from build123d import *

# Parameters (mm, degrees)
BOSS_EXTRUDE1_DEPTH = 35.687
SKETCH2_R           = 4.1656
CUT_EXTRUDE1_DEPTH  = 77.2
SKETCH3_R           = 4.1656
CUT_EXTRUDE2_DEPTH  = 77.2


with BuildPart() as part:
    # Sketch1 → Boss-Extrude1 (new body, symmetric)
    with BuildSketch(Plane.XY):
        with BuildLine():
            Line((0, 0), (0, 76.2))
            ThreePointArc((0, 76.2), (4.490128061, 74.340128061), (6.35, 69.85))
            Line((6.35, 69.85), (6.35, 14.2748))
            ThreePointArc((6.35, 14.2748), (8.67112018, 8.67112018), (14.2748, 6.35))
            Line((14.2748, 6.35), (69.85, 6.35))
            ThreePointArc((69.85, 6.35), (74.340128061, 4.490128061), (76.2, 0))
            Line((76.2, 0), (0, 0))
        make_face()
    extrude(amount=BOSS_EXTRUDE1_DEPTH, both=True)

    # Sketch2 → Cut-Extrude1 (cut, through all)
    with BuildSketch(Plane(origin=(0, 0, 0), x_dir=(1, 0, 0), z_dir=(0, 1, 0))):
        with Locations((19.05, -19.05)):
            Circle(SKETCH2_R)
        with Locations((57.15, -19.05)):
            Circle(SKETCH2_R)
        with Locations((19.05, 19.05)):
            Circle(SKETCH2_R)
        with Locations((57.15, 19.05)):
            Circle(SKETCH2_R)
    extrude(amount=CUT_EXTRUDE1_DEPTH, mode=Mode.SUBTRACT)

    # Sketch3 → Cut-Extrude2 (cut, through all)
    with BuildSketch(Plane(origin=(0, 0, 0), x_dir=(0, 0, -1), z_dir=(1, 0, 0))):
        with Locations((-19.05, 19.05)):
            Circle(SKETCH3_R)
        with Locations((-19.05, 57.15)):
            Circle(SKETCH3_R)
        with Locations((19.05, 19.05)):
            Circle(SKETCH3_R)
        with Locations((19.05, 57.15)):
            Circle(SKETCH3_R)
    extrude(amount=CUT_EXTRUDE2_DEPTH, mode=Mode.SUBTRACT)


solid = part.part
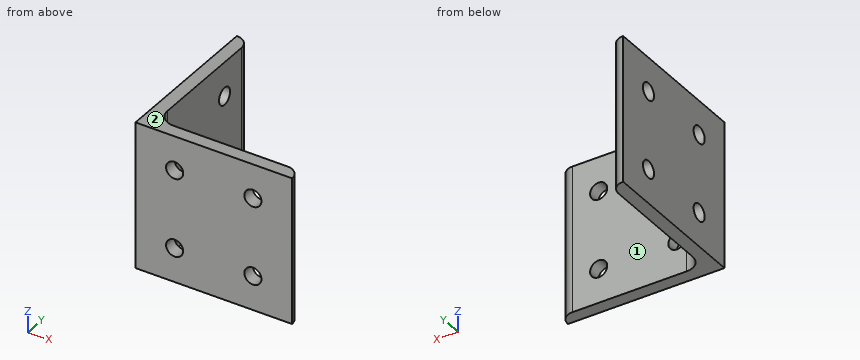
Here's how the part is built. I have some questions about the finished solid (model axes, mm). Face numbers are marked on the shaded views. A direction names the side the tool comes from. Round coordinates to 2 decimals unless told otherwise and drop trailing zeros. Order: outer loops, then holes, each group sorted by start corner. A loop starts at its lowest first (then second) coordinate and runs counter-clockwise, first axis right, second up. Notation, with made-up numbers: M -40,84 L -35,84 A6 ccw -35,88 Z; hole C 31,7 d1. An arc over 180 degrees is marked long. Return JSON: item names as keys, results as strings. Group by question number.
1. If we section it at C-C on z = -19.05: List the corners of the cut face in (x, y) for me, then the cut area to 3 significant figures.
2. On a 3-axis mill with a long thin cutter (end or side, diameter ignored), from which of +Z, -Z, +X, -X, +Y, -Y can I reach the whole of each face in a straight line? I mean the marked faces 1 and 2. Say none if no direction works.
3. Please list where these lines run through material, in increasing order: probe 1 along Z at (x, y) = (5, 57); probe 2 along Y at (x, z) = (4, -19).
4. If we section it at A-A on x = 19.05: List the corners of the cut face in (y, z) for me, then the cut area to 3 significant figures.
5. I'm going to push flat-ended pins straight in: pin 1 Ø7.5 at (y, z) = (19.05, -19.05) entering from +X; pin 2 Ø9.5 at (y, z) = (19.05, 19.05) entering from -X; pin 3 Ø13.5 at (x, z) = (19.05, -19.05) entering from +Y; pin 4 Ø11 at (y, z) = (57.15, 19.05) entering from +X. Where does each tip first touch, or does it pass through?
6. If we section it at D-D on z = -28.5: List the corners of the cut face in (x, y) for me.
Reply:
{
 "1": {"outline": "M 0,0 L 14.88,0 L 14.88,6.35 L 14.27,6.35 A7.92 cw 6.35,14.27 L 6.35,14.88 L 0,14.88 Z; M 0,23.22 L 6.35,23.22 L 6.35,52.98 L 0,52.98 Z; M 0,61.32 L 6.35,61.32 L 6.35,69.85 A6.35 ccw 0,76.2 Z; M 23.22,0 L 52.98,0 L 52.98,6.35 L 23.22,6.35 Z; M 61.32,0 L 76.2,0 A6.35 ccw 69.85,6.35 L 61.32,6.35 Z", "area": "712 mm^2"},
 "2": {"face 1": "+Z, -Z, +X, +Y", "face 2": "+Z, +X, -X, +Y, -Y"},
 "3": {"probe 1": "-35.69 to -23.21, -14.89 to 14.89, 23.21 to 35.69", "probe 2": "0 to 14.88, 23.22 to 52.98, 61.32 to 74.78"},
 "4": {"outline": "M 0,-35.69 L 6.35,-35.69 L 6.35,-23.22 L 0,-23.22 Z; M 0,-14.88 L 6.35,-14.88 L 6.35,14.88 L 0,14.88 Z; M 0,23.22 L 6.35,23.22 L 6.35,35.69 L 0,35.69 Z", "area": "347 mm^2"},
 "5": {"pin 1": "through", "pin 2": "x = 0", "pin 3": "y = 6.6", "pin 4": "x = 6.35"},
 "6": {"outline": "M 0,0 L 76.2,0 A6.35 ccw 69.85,6.35 L 14.27,6.35 A7.92 cw 6.35,14.27 L 6.35,69.85 A6.35 ccw 0,76.2 Z"}
}
